from build123d import *

# Parameters (mm, degrees)
BOSS_EXTRUDE1_DEPTH = 19
BOSS_EXTRUDE2_DEPTH = 60
CUT_EXTRUDE1_DEPTH  = 29
SKETCH4_R           = 4.5
CUT_EXTRUDE2_DEPTH  = 61


with BuildPart() as part:
    # Sketch1 → Boss-Extrude1 (new body, symmetric)
    with BuildSketch(Plane.XY):
        with BuildLine():
            Line((-36, 0), (-27, 0))
            ThreePointArc((-27, 0), (0, 27), (27, 0))
            Line((27, 0), (36, 0))
            ThreePointArc((36, 0), (0, 36), (-36, 0))
        make_face()
    extrude(amount=BOSS_EXTRUDE1_DEPTH, both=True)

    # Sketch2 → Boss-Extrude2 (add)
    with BuildSketch(Plane(origin=(0, 60, 0), x_dir=(-1, 0, 0), z_dir=(0, -1, 0))):
        with BuildLine():
            Line((-38, 9), (38, 9))
            ThreePointArc((38, 9), (47, 0), (38, -9))
            Line((38, -9), (-38, -9))
            ThreePointArc((-38, -9), (-47, 0), (-38, 9))
        make_face()
    extrude(amount=BOSS_EXTRUDE2_DEPTH)

    # Sketch3 → Cut-Extrude1 (cut, through all)
    with BuildSketch(Plane.XY.offset(9)):
        with BuildLine():
            Line((-27, 0), (27, 0))
            ThreePointArc((27, 0), (0, 27), (-27, 0))
        make_face()
    extrude(amount=-CUT_EXTRUDE1_DEPTH, mode=Mode.SUBTRACT)

    # Sketch4 → Cut-Extrude2 (cut, through all)
    with BuildSketch(Plane.XZ):
        with Locations((-38, 0)):
            Circle(SKETCH4_R)
        with Locations((38, 0)):
            Circle(SKETCH4_R)
    extrude(amount=-CUT_EXTRUDE2_DEPTH, mode=Mode.SUBTRACT)


solid = part.part
Here's how the part is built. I have some questions about the finished solid (model axes, mm). A direction names the side the tool comes from. Give positions to 0.01 mm unless a question says otherwise; leave off trailing zeros. Loops run counter-clockwise (first coordinate to the right, second up) from the corner with the lowest first, then second, coordinate; pieces in that order, holes last. Notation, with made-up numbers: (62, 74) -> (106, 74) arc R25 ccw to (106, 91) -> close; hole circle Ø7 at (68, 37). An arc over 180 degrees is marked (long way). One line per item, written item: value.
Q1. If I drill on line 1 along Z through (x, y) = (-38, 41); line 2 along X through (y, z) = (22, 1.5); line 3 along Z through (x, y) = (23, 47), over which ranges is the centre line in solid material (lowest first)?
Answers follow:
line 1: -9 to -4.5, 4.5 to 9
line 2: -46.87 to -42.24, -33.76 to -15.65, 15.65 to 33.76, 42.24 to 46.87
line 3: -9 to 9
Q2. I'm going to push flat-ended pins straight in: pin 1 Ø6 at (y, z) = (32.5, -4) entering from +X; pin 2 Ø2 at (y, z) = (28.5, 11) entering from -X; pin 3 Ø2 at (x, z) = (12.5, 8.5) entering from -Y; pin 4 Ø5.5 at (x, z) = (-38, 0) entering from +Y. Where does each tip first touch, or does it pass through?
Answers follow:
pin 1: x = 46.94
pin 2: x = -23.23
pin 3: y = 23.38
pin 4: through
Q3. We'd pull the mould along X, two halves only. Please class faces 3 (the face through (-0.594, 26.993, 0.266)), 4 (the face through (-1, 60, 0)), 5 (the face through (0.79, 35.99, 14.07)), 6 (the face through (-33.708, 29.58, 1.352)): pulls with the +X half, pulls with the -X half, needs draft (parallel to the pull), parting line crosses it, or undercut.
Answers follow:
face 3: undercut
face 4: needs draft
face 5: parting line crosses it
face 6: undercut
Q4. Suppose I cut it at A-A on y = 4.5. Please give me the cut outline in (x, z).
Answers follow:
outline: (-38, -9) -> (-35.72, -9) -> (-35.72, -19) -> (-26.62, -19) -> (-26.62, 19) -> (-35.72, 19) -> (-35.72, 9) -> (-38, 9) arc R9 ccw to start; (26.62, -19) -> (35.72, -19) -> (35.72, -9) -> (38, -9) arc R9 ccw to (38, 9) -> (35.72, 9) -> (35.72, 19) -> (26.62, 19) -> close; hole circle Ø9 at (-38, 0); hole circle Ø9 at (38, 0)
Q5. On a 3-axis mill with a long thin cutter (end or side, diameter ignored), from which of +Z, -Z, +X, -X, +Y, -Y can I reach the whole of each face in a straight line? I mean faces 1 (the face through (-1, 30, -19)), 2 (the face through (0.79, 35.99, -13.93)). Say none if no direction works.
Answers follow:
face 1: -Z, +X, -X, +Y, -Y
face 2: -Z, +Y
Q6. Suppose I cut it at B-B on z = 0. Please give me the cut outline in (x, y).
Answers follow:
outline: (-47, 0) -> (-42.5, 0) -> (-42.5, 60) -> (-47, 60) -> close; (-33.5, 0) -> (-27, 0) arc R27 cw to (27, 0) -> (33.5, 0) -> (33.5, 60) -> (-33.5, 60) -> close; (42.5, 0) -> (47, 0) -> (47, 60) -> (42.5, 60) -> close
Q7. Suppose I cut it at C-C on x = 0. Please give me the cut outline in (y, z).
Answers follow:
outline: (27, -19) -> (36, -19) -> (36, -9) -> (60, -9) -> (60, 9) -> (36, 9) -> (36, 19) -> (27, 19) -> close
Q8. Suppose I cut it at D-D on z = 8. Please give me the cut outline in (x, y), then the cut area to 3 significant figures.
Answers follow:
outline: (-42.12, 0) -> (-27, 0) arc R27 cw to (27, 0) -> (42.12, 0) -> (42.12, 60) -> (-42.12, 60) -> close
area: 3,910 mm^2
